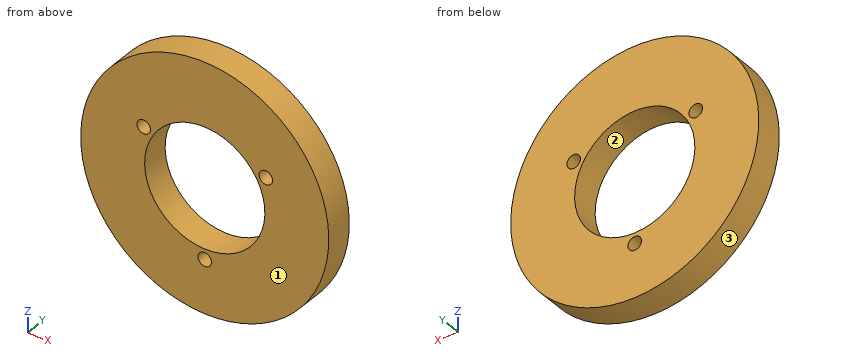
from build123d import *

# Parameters (mm, degrees)
SKETCH1_R           = 41.91
SKETCH1_R_2         = 20.32
BOSS_EXTRUDE1_DEPTH = 9.525
SKETCH2_R           = 2.286
CUT_EXTRUDE1_DEPTH  = 61.030174288


with BuildPart() as part:
    # Sketch1 → Boss-Extrude1 (new body)
    with BuildSketch(Plane(origin=(0, 0, 0), x_dir=(1, 0, 0), z_dir=(0, 1, 0))):
        with Locations(Location((0, 0, 0), (0, 0, 90))):
            Circle(SKETCH1_R)
        with Locations(Location((0, 0, 0), (0, 0, 90))):
            Circle(SKETCH1_R_2, mode=Mode.SUBTRACT)
    extrude(amount=BOSS_EXTRUDE1_DEPTH)

    # Sketch2 → Cut-Extrude1 (cut, through all)
    with BuildSketch(Plane(origin=(0, 9.525, 0), x_dir=(1, 0, 0), z_dir=(0, 1, 0))):
        with Locations(Location((0, 23.8125, 0), (0, 0, 270))):
            Circle(SKETCH2_R)
        with Locations(Location((20.622229928, -11.90625, 0), (0, 0, 270))):
            Circle(SKETCH2_R)
        with Locations(Location((-20.622229928, -11.90625, 0), (0, 0, 270))):
            Circle(SKETCH2_R)
    extrude(amount=-CUT_EXTRUDE1_DEPTH, mode=Mode.SUBTRACT)


solid = part.part
Read the model definition and answer for the solid it produces. Units are mm, in the model's axes. Face numbers are marked on the shaded views. Round coordinates to 2 decimals unless told otherwise and drop trailing zeros. Write each loop counter-clockwise with the first axis right and the second up, starting at its lowest first coordinate (ties: lowest second). Pieces come first, ordered by that corner, then holes. Notation, with made-up numbers: (-3, 81.5) - (18, 81.5) arc R28 cw to (18, 118.5) - close; hole circle Ø9 at (45, 2). An arc over 180 degrees is marked (long way). Use a Markdown table: item, result.
(1) The part is cut by section A-A (x = 0). Write down the section's boundary in (y, z) (1 decimal), then the cut area to 3 significant figures.
Reported:
| item | result |
|---|---|
| outline | (0, -41.9) - (9.5, -41.9) - (9.5, -26.1) - (0, -26.1) - close; (0, -21.5) - (9.5, -21.5) - (9.5, -20.3) - (0, -20.3) - close; (0, 20.3) - (9.5, 20.3) - (9.5, 41.9) - (0, 41.9) - close |
| area | 368 mm2 |
(2) Straight lines are drawn through the part: line 1 along X through (y, z) = (7, 0); line 2 along Z through (x, y) = (-12.5, 1); line 3 along X through (y, z) = (1.25, 2.5). For each, find the intervals that lie inside material, in ascending order. Write a range as [from, to].
Reported:
| item | result |
|---|---|
| line 1 | [-41.91, -20.32], [20.32, 41.91] |
| line 2 | [-40, -16.02], [16.02, 40] |
| line 3 | [-41.84, -20.17], [20.17, 41.84] |
(3) The mould has two halves that part along X. Classify the marked faces 1, 2 and 3: released by +X, released by -X, zero draft, split by the parting line, or undercut.
Reported:
| item | result |
|---|---|
| face 1 | zero draft |
| face 2 | undercut |
| face 3 | split by the parting line |
(4) Each of these flat-tipped pins is pushed along its axis until it touches: pin 1 Ø3 at (x, y) = (20.5, 3) entering from -Z; pin 2 Ø4 at (x, z) = (0, -23.81) entering from -Y; pin 3 Ø5 at (y, z) = (2.5, 13) entering from +X; pin 4 Ø2 at (x, y) = (8, 8) entering from +Z. Where does it stop, or does it pass through?
Reported:
| item | result |
|---|---|
| pin 1 | z = -37.36 |
| pin 2 | through |
| pin 3 | x = 40.57 |
| pin 4 | z = 41.32 |
(5) The part is cut by section B-B (z = 0). Write down the section's boundary in (x, y) (3 decimals), then the cut area to 3 significant figures.
Reported:
| item | result |
|---|---|
| outline | (-41.91, 0) - (-20.32, 0) - (-20.32, 9.525) - (-41.91, 9.525) - close; (20.32, 0) - (41.91, 0) - (41.91, 9.525) - (20.32, 9.525) - close |
| area | 411 mm2 |
(6) The part is cut by section C-C (y = 1.5). Write down the section's boundary in (x, z), then the cut area to 3 significant figures.
Reported:
| item | result |
|---|---|
| outline | circle Ø83.82 at (0, 0); hole circle Ø4.57 at (-20.62, 11.91); hole circle Ø40.64 at (0, 0); hole circle Ø4.57 at (0, -23.81); hole circle Ø4.57 at (20.62, 11.91) |
| area | 4,170 mm2 |
(7) The part is cut by section D-D (z = 16). Write down the section's boundary in (x, y) (3 decimals), then the cut area to 3 significant figures.
Reported:
| item | result |
|---|---|
| outline | (-38.736, 0) - (-12.526, 0) - (-12.526, 9.525) - (-38.736, 9.525) - close; (12.526, 0) - (38.736, 0) - (38.736, 9.525) - (12.526, 9.525) - close |
| area | 499 mm2 |
